Build history of the part. All positions in model axes, mm. A direction names the side the tool comes from. Round coordinates to 2 decimals unless told otherwise and drop trailing zeros. Write each loop counter-clockwise with the first axis right and the second up, starting at its lowest first coordinate (ties: lowest second). Pieces come first, ordered by that corner, then holes. Notation, with made-up numbers: M 16,65.25 L 49,65.25 A10 cw 49,69.25 Z; hole C 53.5,86 d9. An arc over 180 degrees is marked long. One line per item, written item: value. Start each with the question number.
```python
from build123d import *

# Parameters (mm, degrees)
SKETCH1_R           = 2
BOSS_EXTRUDE1_DEPTH = 37.338
SKETCH2_R           = 3.5
BOSS_EXTRUDE2_DEPTH = 2.54
CHAMFER1_SIZE       = 0.254
CHAMFER2_SIZE       = 0.254
CHAMFER3_SIZE       = 0.254


with BuildPart() as part:
    # Sketch1 → Boss-Extrude1 (new body)
    with BuildSketch(Plane(origin=(0, 0, 0), x_dir=(1, 0, 0), z_dir=(0, 1, 0))):
        with Locations(Location((0, 0, 0), (0, 0, 270))):
            Circle(SKETCH1_R)
    extrude(amount=BOSS_EXTRUDE1_DEPTH)

    # Sketch2 → Boss-Extrude2 (add)
    with BuildSketch(Plane.XZ):
        with Locations(Location((0, 0, 0), (0, 0, 270))):
            Circle(SKETCH2_R)
    extrude(amount=BOSS_EXTRUDE2_DEPTH)

    # Chamfer1
    chamfer1_edges = [part.edges().sort_by_distance(p)[0] for p in [
        (0, -2.54, 3.5),
    ]]
    chamfer(chamfer1_edges, length=CHAMFER1_SIZE)

    # Chamfer2
    chamfer2_edges = [part.edges().sort_by_distance(p)[0] for p in [
        (0, 37.338, -2),
    ]]
    chamfer(chamfer2_edges, length=CHAMFER2_SIZE)

    # Chamfer3
    chamfer3_edges = [part.edges().sort_by_distance(p)[0] for p in [
        (0, 0, 3.5),
    ]]
    chamfer(chamfer3_edges, length=CHAMFER3_SIZE)


solid = part.part
```
Item 1: Cut at B-B, the plane z = 0. Write the cut outline in (x, y), plus the area to 3 significant figures.
Item 2: Cut at C-C, the plane y = 29. Write the cut outline in (x, z).
Item 3: Cut at A-A, the plane x = 0. Write the cut outline in (y, z).
Item 4: Which spindle directions (+Z, -Z, +X, -X, +Y, -Y) get a long thin tool onto all of the face, cutting with end or side? Do faces 1 (the flat face through (-2, 0, -1)), 2 (the cylindrical face through (-3.417, -1.256, 0.759)). Say none if no direction does.
Item 5: Drop flat-ended pins along their axis: pin 1 (4 mm diameter, centred on y = 27.5, z = 0, fed in from -X); pin 2 (3 mm diameter, centred on x = 1.5, y = 19.5, fed in from -Z); pin 3 (4 mm diameter, centred on x = -1, z = 1.5, fed in from +Y); pin 4 (1.5 mm diameter, centred on x = 1, y = 16, fed in from +Z). Give the stop position or say it passes through.
Item 6: Drill centre lines: line 1 (Y direction, x = -3, z = 0.25); line 2 (Z direction, x = -1.25, y = 31); line 3 (X direction, y = 35, z = 0.75). Where is each one in solid material? Low to high.
Computed values:
1. outline: M -3.5,-2.29 L -3.25,-2.54 L 3.25,-2.54 L 3.5,-2.29 L 3.5,-0.25 L 3.25,0 L 2,0 L 2,37.08 L 1.75,37.34 L -1.75,37.34 L -2,37.08 L -2,0 L -3.25,0 L -3.5,-0.25 Z
1. area: 167 mm2
2. outline: C 0,0 d4
3. outline: M -2.54,-3.25 L -2.29,-3.5 L -0.25,-3.5 L 0,-3.25 L 0,-2 L 37.08,-2 L 37.34,-1.75 L 37.34,1.75 L 37.08,2 L 0,2 L 0,3.25 L -0.25,3.5 L -2.29,3.5 L -2.54,3.25 Z
4. face 1: +Y
4. face 2: +Y, -Y
5. pin 1: stops at x = -2
5. pin 2: stops at z = -2
5. pin 3: stops at y = 37.34
5. pin 4: stops at z = 1.98
6. line 1: y = -2.54 to 0
6. line 2: z = -1.56 to 1.56
6. line 3: x = -1.85 to 1.85
